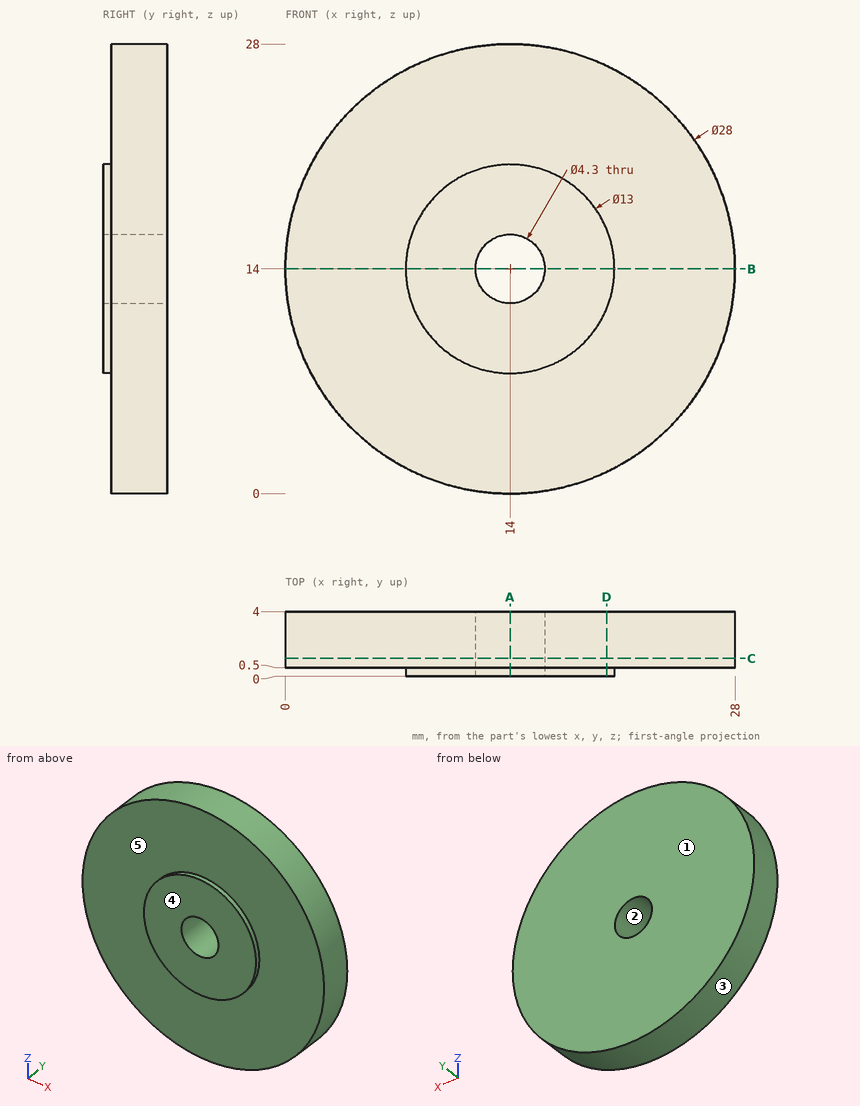
Answer from the drawing. Dimensions are ordinates in mm from the lowest x, y and z of the part. A direction names the side the tool comes from. Give positions to 0.01 mm unless a question says otherwise; leave off trailing zeros. Loops run counter-clockwise (first coordinate to the right, second up) from the corner with the lowest first, then second, coordinate; pieces in that order, holes last.
Item 1: The mould has two halves that part along Z. Classify the marked faces 1, 2 and 3: released by +Z, released by -Z, zero draft, split by the parting line, or undercut.
Item 2: The part is cut by section B-B (z = 14). Write down the section's boundary in (x, y).
Item 3: The part is cut by section C-C (y = 1.1). Write down the section's boundary in (x, z).
Item 4: The part is cut by section D-D (x = 20). Write down the section's boundary in (y, z), and give its area (3 significant figures).
Item 5: Each of these flat-tipped pins is pushed along its axis until it touches: pin 1 Ø2.5 at (x, z) = (14, 14) entering from +Y; pin 2 Ø1.5 at (y, z) = (1.5, 10.5) entering from -X. Where does it stop, or does it pass through?
Item 6: For the marked faces 4 and 5, determine the directions among +Z, -Z, +X, -X, +Y, -Y from which every point of the face is accessible in a straight line to the end or side of a thin tool.
Item 7: The part is cut by section A-A (x = 14). Write down the section's boundary in (y, z), and give its area (3 significant figures).
Item 8: Find the intervals of material crossed by line 1 along X through (y, z) = (1.6, 14); line 2 along Y through (x, z) = (1.5, 13.25), in increasing order.
Taken from the geometry:
1. face 1: zero draft
1. face 2: undercut
1. face 3: split by the parting line
2. outline: (0, 0.5) - (7.5, 0.5) - (7.5, 0) - (11.85, 0) - (11.85, 4) - (0, 4) - close; (16.15, 0) - (20.5, 0) - (20.5, 0.5) - (28, 0.5) - (28, 4) - (16.15, 4) - close
3. outline: circle Ø28 at (14, 14); hole circle Ø4.3 at (14, 14)
4. outline: (0, 11.5) - (0.5, 11.5) - (0.5, 1.35) - (4, 1.35) - (4, 26.65) - (0.5, 26.65) - (0.5, 16.5) - (0, 16.5) - close
4. area: 91.0 mm2
5. pin 1: passes through
5. pin 2: stops at x = 0.27
6. face 4: +Z, -Z, +X, -X, -Y
6. face 5: -Y
7. outline: (0, 7.5) - (0.5, 7.5) - (0.5, 0) - (4, 0) - (4, 11.85) - (0, 11.85) - close; (0, 16.15) - (4, 16.15) - (4, 28) - (0.5, 28) - (0.5, 20.5) - (0, 20.5) - close
7. area: 87.3 mm2
8. line 1: x = 0 to 11.85, 16.15 to 28
8. line 2: y = 0.5 to 4
